Build history of the part. All positions in model axes, mm. Face numbers are marked on the shaded views. A direction names the side the tool comes from. Round coordinates to 2 decimals unless told otherwise and drop trailing zeros. Loops run counter-clockwise (first coordinate to the right, second up) from the corner with the lowest first, then second, coordinate; pieces in that order, holes last. Notation, with made-up numbers: (68, 86) -> (108, 86) arc R11 cw to (108, 105) -> close; hole circle Ø2 at (35, 53.25). An arc over 180 degrees is marked (long way). Put each result on its own line as item: value. Start each with the question number.
```python
from build123d import *

# Parameters (mm, degrees)
BOSS_EXTRUDE1_DEPTH = 6
FILLET1_R           = 1
SKETCH2_R           = 16
BOSS_EXTRUDE2_DEPTH = 2
CHAMFER1_SIZE       = 1
CHAMFER1_SIZE2      = 1.732050808
SKETCH3_R           = 3.5
CUT_EXTRUDE1_DEPTH  = 9


with BuildPart() as part:
    # Sketch1 → Boss-Extrude1 (new body)
    with BuildSketch(Plane(origin=(0, 0, 0), x_dir=(1, 0, 0), z_dir=(0, 1, 0))):
        with BuildLine():
            Line((-18, 22.5), (24, 22.5))
            ThreePointArc((24, 22.5), (26.828427125, 21.328427125), (28, 18.5))
            Line((28, 18.5), (28, -18.5))
            ThreePointArc((28, -18.5), (26.828427125, -21.328427125), (24, -22.5))
            Line((24, -22.5), (-18, -22.5))
            ThreePointArc((-18, -22.5), (-20.828427125, -21.328427125), (-22, -18.5))
            Line((-22, -18.5), (-22, 18.5))
            ThreePointArc((-22, 18.5), (-20.828427125, 21.328427125), (-18, 22.5))
        make_face()
    extrude(amount=BOSS_EXTRUDE1_DEPTH)

    # Fillet1
    fillet1_edges = [part.edges().sort_by_distance(p)[0] for p in [
        (-20.828427125, 6, -21.328427125),
        (-22, 6, 0),
        (-20.828427125, 6, 21.328427125),
        (3, 6, 22.5),
        (26.828427125, 6, 21.328427125),
        (28, 6, 0),
        (26.828427125, 6, -21.328427125),
        (3, 6, -22.5),
    ]]
    fillet(fillet1_edges, radius=FILLET1_R)

    # Sketch2 → Boss-Extrude2 (add)
    with BuildSketch(Plane.XZ):
        Circle(SKETCH2_R)
    extrude(amount=BOSS_EXTRUDE2_DEPTH)

    # Chamfer1
    chamfer1_edges = [part.edges().sort_by_distance(p)[0] for p in [
        (-16, -2, 0),
    ]]
    chamfer1_side = [part.faces().sort_by_distance(p)[0] for p in [
        (-16, -1, 0),
    ]]
    chamfer(chamfer1_edges, length=CHAMFER1_SIZE, length2=CHAMFER1_SIZE2, reference=chamfer1_side[0])

    # Sketch3 → Cut-Extrude1 (cut, through all)
    with BuildSketch(Plane(origin=(0, 6, 0), x_dir=(1, 0, 0), z_dir=(0, 1, 0))):
        with Locations((-16.263455967, 16.263455967)):
            Circle(SKETCH3_R)
        with Locations((16.263455967, 16.263455967)):
            Circle(SKETCH3_R)
        with Locations((16.263455967, -16.263455967)):
            Circle(SKETCH3_R)
        with Locations((-16.263455967, -16.263455967)):
            Circle(SKETCH3_R)
    extrude(amount=-CUT_EXTRUDE1_DEPTH, mode=Mode.SUBTRACT)


solid = part.part
```
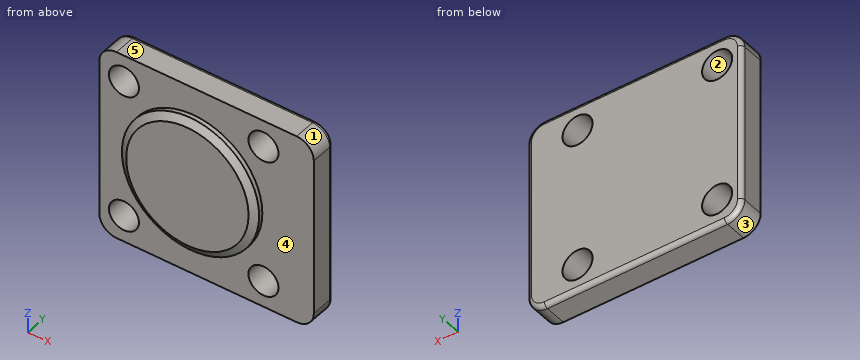
Item 1: Pull direction X, two halves, no side cores. Call the marked faces 1, 2 and 3: +X half, -X half, draft (parallel to the pull), parting line (faces both ways), or undercut.
Item 2: Wall check: line 1 (X direction, y = 5.5, z = 19); line 2 (Z direction, x = 15.5, y = 5.25); line 3 (X direction, y = 3.75, z = -15). Give the ranges that are in metal, low to high. Write a range as from..to.
Item 3: Cut at D-D on z = 0. Write the cut outline in (x, y), then the cut area to 3 significant figures.
Item 4: Drop flat-ended pins along their axis: pin 1 (11 mm diameter, centred on x = -16.26, z = -16.26, fed in from +Y); pin 2 (1.5 mm diameter, centred on y = -1, z = -14, fed in from +X). Give the stop position or say it passes through.
Item 5: Cut at A-A on z = 17.5. Write the cut outline in (x, y).
Item 6: Cut at C-C on x = 0. Write the cut outline in (y, z), then the cut area to 3 significant figures.
Item 7: Cut at B-B on y = 3.5. Write the cut outline in (x, z), then the cut area to 3 significant figures.
Item 8: 3-axis set-ups, long thin cutter, end or side, ignore diameter. For the marked faces 4 and 5: which of +Z, -Z, +X, -X, +Y, -Y reach the whole face in a straight line?
Ans:
1. face 1: +X half
1. face 2: undercut
1. face 3: -X half
2. line 1: x = -21.83..-18.45, -14.08..14.08, 18.45..27.83
2. line 2: z = -22.47..-19.68, -12.85..12.85, 19.68..22.47
2. line 3: x = -22..-19.53, -13..13, 19.53..28
3. outline: (-22, 0) -> (-16, 0) -> (-16, -1) -> (-14.27, -2) -> (14.27, -2) -> (16, -1) -> (16, 0) -> (28, 0) -> (28, 5) arc R1 ccw to (27, 6) -> (-21, 6) arc R1 ccw to (-22, 5) -> close
3. area: 362 mm2
4. pin 1: stops at y = 6
4. pin 2: stops at x = 8.97
5. outline: (-22, 0) -> (-19.54, 0) -> (-19.54, 6) -> (-21, 6) arc R1 ccw to (-22, 5) -> close; (-12.99, 0) -> (12.99, 0) -> (12.99, 6) -> (-12.99, 6) -> close; (19.54, 0) -> (28, 0) -> (28, 5) arc R1 ccw to (27, 6) -> (19.54, 6) -> close
6. outline: (-2, -14.27) -> (-1, -16) -> (0, -16) -> (0, -22.5) -> (5, -22.5) arc R1 ccw to (6, -21.5) -> (6, 21.5) arc R1 ccw to (5, 22.5) -> (0, 22.5) -> (0, 16) -> (-1, 16) -> (-2, 14.27) -> close
6. area: 332 mm2
7. outline: (-22, -18.5) arc R4 ccw to (-18, -22.5) -> (24, -22.5) arc R4 ccw to (28, -18.5) -> (28, 18.5) arc R4 ccw to (24, 22.5) -> (-18, 22.5) arc R4 ccw to (-22, 18.5) -> close; hole circle Ø7 at (-16.26, -16.26); hole circle Ø7 at (-16.26, 16.26); hole circle Ø7 at (16.26, -16.26); hole circle Ø7 at (16.26, 16.26)
7. area: 2,080 mm2
8. face 4: -Y
8. face 5: +Z, +X, -X, +Y, -Y
